```python
from build123d import *

# Parameters (mm, degrees)
SKETCH1_R           = 4.49961
SKETCH1_R_2         = 1.9939
BOSS_EXTRUDE1_DEPTH = 6.35
FILLET2_R           = 3.175


with BuildPart() as part:
    # Sketch1 → Boss-Extrude1 (new body)
    with BuildSketch(Plane.XY):
        with BuildLine():
            Line((-83.400738686, -3.175), (-5.499261314, -3.175))
            ThreePointArc((-5.499261314, -3.175), (2.532857004, -5.822983376), (6.072024587, 1.858229644))
            ThreePointArc((6.072024587, 1.858229644), (6.667791277, 4.818557399), (9.470894014, 5.941541551))
            Line((9.470894014, 5.941541551), (83.073913127, -2.525710148))
            ThreePointArc((83.073913127, -2.525710148), (95.20839431, -0.725714286), (83.799627413, 3.782684163))
            Line((83.799627413, 3.782684163), (10.196608307, 12.249935861))
            ThreePointArc((10.196608307, 12.249935861), (4.237192952, 10.972727963), (0.272052538, 6.344169561))
            ThreePointArc((0.272052538, 6.344169561), (-3.056441857, 5.566027594), (-5.499261314, 3.175))
            Line((-5.499261314, 3.175), (-83.400738686, 3.175))
            ThreePointArc((-83.400738686, 3.175), (-95.25, 0), (-83.400738686, -3.175))
        make_face()
        with Locations((-88.9, 0)):
            Circle(SKETCH1_R, mode=Mode.SUBTRACT)
        Circle(SKETCH1_R_2, mode=Mode.SUBTRACT)
        with Locations((88.9, 0)):
            Circle(SKETCH1_R, mode=Mode.SUBTRACT)
    extrude(amount=BOSS_EXTRUDE1_DEPTH)

    # Fillet2
    fillet2_edges = [part.edges().sort_by_distance(p)[0] for p in [
        (-5.499261314, -3.175, 3.175),
        (-83.400738686, -3.175, 3.175),
        (-83.400738686, 3.175, 3.175),
        (-5.499261314, 3.175, 3.175),
        (0.272052538, 6.344169561, 3.175),
        (83.799627413, 3.782684163, 3.175),
        (83.073913127, -2.525710148, 3.175),
    ]]
    fillet(fillet2_edges, radius=FILLET2_R)


solid = part.part
```
Model file for the job. Use its own axes, mm. A direction names the side the tool comes from. Round coordinates to 2 decimals unless told otherwise and drop trailing zeros. Order: outer loops, then holes, each group sorted by start corner. A loop starts at its lowest first (then second) coordinate and runs counter-clockwise, first axis right, second up. Notation, with made-up numbers: (42.25, -13.5) -> (99.25, -13.5) arc R31 ccw to (99.25, 19.5) -> close; hole circle Ø2 at (0, 71). An arc over 180 degrees is marked (long way). Use one line per item in the form item = value.
Item 1: Tool access for faces 1 (the face through (-93.395, 0.198, 3.131)), 2 (the face through (-45, -3.175, 3)), 3 (the face through (-44, 3.175, 3)): list every direction of +Z, -Z, +X, -X, +Y, -Y with a clear straight run to the whole face (end or side of a thin tool).
Returned:
face_1 = +Z, -Z
face_2 = +Z, -Z, -Y
face_3 = +Z, -Z, +Y
Item 2: Drill centre lines: line 1 (Y direction, x = -88.9, z = 2.5); line 2 (X direction, y = -3, z = 5.5); line 3 (Y direction, x = -27, z = 5.75) (3 decimals). Where is each one in solid material? Low to high.
Returned:
line_1 = -6.35 to -4.5, 4.5 to 6.35
line_2 = -94.5 to -92.25, -85.55 to 5.6, 83.08 to 85.55, 92.25 to 94.5
line_3 = -3.175 to 3.175
Item 3: Cut at B-B, the plane y = 0. Write the cut outline in (x, z), and give its area (3 significant figures).
Returned:
outline = (-95.25, 0) -> (-93.4, 0) -> (-93.4, 6.35) -> (-95.25, 6.35) -> close; (-84.4, 0) -> (-1.99, 0) -> (-1.99, 6.35) -> (-84.4, 6.35) -> close; (1.99, 0) -> (6.35, 0) -> (6.35, 6.35) -> (1.99, 6.35) -> close; (61.12, 0) -> (84.4, 0) -> (84.4, 6.35) -> (61.12, 6.35) -> close; (93.4, 0) -> (95.25, 0) -> (95.25, 6.35) -> (93.4, 6.35) -> close
area = 722 mm^2
Item 4: Flat gauge pins, fed straight in: pin 1 Ø1 at (y, z) = (-0.5, 4) entering from +X; pin 2 Ø1.5 at (x, z) = (-22.5, 5.5) entering from -Y (3 decimals). Where does each tip first touch, or does it go through?
Returned:
pin_1 = 95.25
pin_2 = -3.175
Item 5: Pull direction Y, two halves, no side cores. Call faces 4 (the face through (1.9, 0.6, 3.1)), 5 (the face through (95.18, -0.94, 3.13)), 6 (the face through (44.973, 1.857, 3.131)): released by +Y, released by -Y, zero draft, split by the parting line, or undercut.
Returned:
face_4 = undercut
face_5 = split by the parting line
face_6 = released by -Y
Item 6: Cut at A-A, the plane x = 88.9. Write the cut outline in (y, z).
Returned:
outline = (-6.35, 0) -> (-4.5, 0) -> (-4.5, 6.35) -> (-6.35, 6.35) -> close; (4.5, 0) -> (6.35, 0) -> (6.35, 6.35) -> (4.5, 6.35) -> close
Item 7: Cut at D-D, the plane x = -68.5. Write the cut outline in (y, z) (3 decimals).
Returned:
outline = (-3.175, 0) -> (3.175, 0) -> (3.175, 6.35) -> (-3.175, 6.35) -> close
Item 8: Cut at C-C, the plane z = 1.25. Give the number of separate pieces and of enclosed holes in the cut face, and give its area (3 significant figures).
Returned:
separate_pieces = 1
enclosed_holes = 3
area = 1,250 mm^2
